```python
from build123d import *

# Parameters (mm, degrees)
F1_DEPTH = 20
F2_W     = 5
F2_H     = 5
F3_DEPTH = 14.204988947
F4_SIZE  = 2.5
F5_R     = 2.5


# Not quite as in the source:
# - a feature names something its author has since deleted; it is built from what else it names


with BuildPart() as f1:
    # F0 (on Top) → F1 (new body)
    with BuildSketch(Plane.XY):
        Polygon((0, -14.203988947), (0, -4.5276075453), (-15, -4.5276075453), (-15, -7.5276075453), (-2.9953992926, -7.5276075453), (-2.9953992926, -11.203988947), (-45, -11.203988947), (-45, -14.203988947), align=None)
    extrude(amount=F1_DEPTH)

    # F2 (on Front) → F3 (cut, through all)
    with BuildSketch(Plane.XZ):
        Polygon((-15, 17.4460405111), (-15, 20), (-20, 20), (-20, 15), (-15, 15), align=None)
        with Locations((-27.5, 17.5)):
            Rectangle(F2_W, F2_H)
        with Locations((-37.5, 17.5)):
            Rectangle(F2_W, F2_H)
    extrude(amount=F3_DEPTH, mode=Mode.SUBTRACT)

    # F4
    f4_edges = [f1.edges().sort_by_distance(p)[0] for p in [
        (-45, -12.703989, 20),
    ]]
    chamfer(f4_edges, length=F4_SIZE)

    # F5
    f5_edges = [f1.edges().sort_by_distance(p)[0] for p in [
        (-15, -4.527608, 10),
    ]]
    fillet(f5_edges, radius=F5_R)


solid = f1.part
```
CAD build for the part. Positions are in the model's coordinates, mm. A direction names the side the tool comes from. Coordinates: 2 decimals unless noted, no trailing zeros. Order: outer loops, then holes, each group sorted by start corner. A loop starts at its lowest first (then second) coordinate and runs counter-clockwise, first axis right, second up. Notation, with made-up numbers: (63.25, 4) -> (91.25, 4) arc R27 ccw to (91.25, 29) -> close; hole circle Ø1 at (-1.5, -19). An arc over 180 degrees is marked (long way). Use one line per item in the form item = value. Start each with the question number.
1) Band-saw the part on B-B on z = 15.5. Give the cut face in (x, y).
2) Band-saw the part on D-D on z = 2.75. Give the cut face in (x, y), then the cut area to 3 significant figures.
3) Drop flat-ended pins along their axis: pin 1 (4 mm diameter, centred on x = -17.5, y = -9.5, fed in from -Z); pin 2 (1.1 mm diameter, centred on y = -9, z = 8.5, fed in from -X); pin 3 (0.9 mm diameter, centred on x = -37.5, y = -12.5, fed in from +Z). Give the stop position or say it passes through.
4) Band-saw the part on A-A on x = -4. Give the cut face in (y, z), then the cut area to 3 significant figures.
5) Band-saw the part on C-C on y = -11.75. Give the cut face in (x, z), then the cut area to 3 significant figures.
6) Pull direction X, two halves, no side cores. Call faces 1 (the flat face through (0, -9, 10)), 2 (the flat face through (-9, -7.528, 10)), 3 (the flat face through (-15, -13, 17)), 4 (the flat face through (-18, -13, 15)): +X half, -X half, draft (parallel to the pull), parting line (faces both ways), or undercut.
7) Tool access for faces 5 (the flat face through (-33, -13, 20)), 6 (the flat face through (-24, -11.204, 10)), 7 (the flat face through (-35, -13, 17)): list every direction of +Z, -Z, +X, -X, +Y, -Y with a clear straight run to the whole face (end or side of a thin tool).
8) Drill centre lines: L1, parallel to Y at x = -9, z = 5.5; L2, parallel to X at y = -10.25, z = 5.5; L3, parallel to Y at x = -18, z = 1.25. Where is each one in solid material? Low to high. Write a range as [from, to].
Entries:
q1.outline = (-45, -14.2) -> (-40, -14.2) -> (-40, -11.2) -> (-45, -11.2) -> close; (-35, -14.2) -> (-30, -14.2) -> (-30, -11.2) -> (-35, -11.2) -> close; (-25, -14.2) -> (-20, -14.2) -> (-20, -11.2) -> (-25, -11.2) -> close; (-15, -14.2) -> (0, -14.2) -> (0, -4.53) -> (-12.5, -4.53) arc R2.5 ccw to (-15, -7.03) -> (-15, -7.53) -> (-3, -7.53) -> (-3, -11.2) -> (-15, -11.2) -> close
q2.outline = (-45, -14.2) -> (0, -14.2) -> (0, -4.53) -> (-12.5, -4.53) arc R2.5 ccw to (-15, -7.03) -> (-15, -7.53) -> (-3, -7.53) -> (-3, -11.2) -> (-45, -11.2) -> close
q2.area = 190 mm2
q3.pin_1 = 0
q3.pin_2 = -3
q3.pin_3 = 15
q4.outline = (-14.2, 0) -> (-11.2, 0) -> (-11.2, 20) -> (-14.2, 20) -> close; (-7.53, 0) -> (-4.53, 0) -> (-4.53, 20) -> (-7.53, 20) -> close
q4.area = 120 mm2
q5.outline = (-45, 0) -> (0, 0) -> (0, 20) -> (-15, 20) -> (-15, 15) -> (-20, 15) -> (-20, 20) -> (-25, 20) -> (-25, 15) -> (-30, 15) -> (-30, 20) -> (-35, 20) -> (-35, 15) -> (-40, 15) -> (-40, 20) -> (-42.5, 20) -> (-45, 17.5) -> close
q5.area = 822 mm2
q6.face_1 = +X half
q6.face_2 = draft
q6.face_3 = undercut
q6.face_4 = undercut
q7.face_5 = +Z, +X, -X, +Y, -Y
q7.face_6 = +Z, -Z, -X
q7.face_7 = +Z, +Y, -Y
q8.L1 = [-14.2, -11.2], [-7.53, -4.53]
q8.L2 = [-3, 0]
q8.L3 = [-14.2, -11.2]
